from build123d import *

# Parameters (mm, degrees)
F0_W     = 127
F0_H     = 90.9382707423
F1_DEPTH = 76.2
F2_W     = 62.1625276506
F2_H     = 90.9382707423
F4_ANGLE = 45
F5_R     = 9.1670821984
F6_DEPTH = 114.3
F7_R     = 6.35


with BuildPart() as f1:
    # F0 (on Top) → F1 (new body)
    with BuildSketch(Plane.XY):
        with Locations((1.3374723494, 2.0061992109)):
            Rectangle(F0_W, F0_H)
    extrude(amount=F1_DEPTH)

    # F2 (on face) → F4 (revolve)
    with BuildSketch(Plane.XY.offset(76.2)):
        with Locations((-31.0812638253, 2.0061992109)):
            Rectangle(F2_W, F2_H)
    revolve(axis=Axis((0, 2.0061992109, 76.2), (0, 1, 0)), revolution_arc=F4_ANGLE)

    # F5 (on face) → F6 (join)
    with BuildSketch(Plane.XY.offset(76.2)):
        with Locations((35.0989550352, -15.1951536536)):
            Circle(F5_R)
    extrude(amount=F6_DEPTH)

    # F7
    f7_edges = [f1.edges().sort_by_distance(p)[0] for p in [
        (-43.955545, 2.006199, 120.155545),
    ]]
    fillet(f7_edges, radius=F7_R)


solid = f1.part
CAD build for the part. Positions are in the model's coordinates, mm. Round coordinates to 2 decimals unless told otherwise and drop trailing zeros. Order: outer loops, then holes, each group sorted by start corner. A loop starts at its lowest first (then second) coordinate and runs counter-clockwise, first axis right, second up. Notation, with made-up numbers: (-38.5, 25) - (-34.5, 25) arc R14 ccw to (-34.5, 46) - close; hole circle Ø5 at (63.25, 34.25). An arc over 180 degrees is marked (long way). Return JSON: item names as keys, results as strings.
(1) Cut at C-C (x = -27). Give the cut face in (y, z).
Answer key:
{"outline": "(-43.46, 0) - (47.48, 0) - (47.48, 103.2) - (-43.46, 103.2) - close"}
(2) Pin check, flat tips, straight feed: pin 1 Ø6 at (x, y) = (4, 28.5) entering from +Z; pin 2 Ø1.5 at (x, z) = (43, 135) entering from -Y; pin 3 Ø10 at (x, z) = (38, 120) entering from -Y. Stop position of each tip, or through.
Answer key:
{"pin 1": "stops at z = 76.2", "pin 2": "stops at y = -20.93", "pin 3": "stops at y = -24.36"}
(3) Pull direction X, two halves, no side cores. Call faces 1 (the face through (27.82, -20.77, 132.55)), 2 (the face through (64.837, 1, 38)), 3 (the face through (-58.79, 2.64, 96.4)), 4 (the face through (-19.9, 2.6, 96.1)): +X half, -X half, draft (parallel to the pull), parting line (faces both ways), or undercut.
Answer key:
{"face 1": "undercut", "face 2": "+X half", "face 3": "-X half", "face 4": "undercut"}
(4) Cut at D-D (y = -21). Give the cut face in (x, z), then the cut area to 3 significant figures.
Answer key:
{"outline": "(-62.16, 0) - (64.84, 0) - (64.84, 76.2) - (42.19, 76.2) - (42.19, 190.5) - (28, 190.5) - (28, 76.2) - (0, 76.2) - (-39.21, 115.41) arc R6.35 ccw to (-48.67, 114.87) arc R62.16 ccw to (-62.16, 76.2) - close", "area": "12,800 mm^2"}
(5) Wall check: probe 1 along Z at (x, y) = (5, 7); probe 2 along X at (y, z) = (-18, 107.5); probe 3 along X at (y, z) = (-28, 114). Give the ranges that are in metal, low to high. Write a range as from..to.
Answer key:
{"probe 1": "z = 0..76.2", "probe 2": "x = -53.71..-31.3, 26.37..43.83", "probe 3": "x = -49.35..-37.8"}
(6) Cut at B-B (z = 85). Give the cut face in (x, y), then the cut area to 3 significant figures.
Answer key:
{"outline": "(-61.54, -43.46) - (-8.8, -43.46) - (-8.8, 47.48) - (-61.54, 47.48) - close; circle Ø18.33 at (35.1, -15.2)", "area": "5,060 mm^2"}
(7) Cut at A-A (y = 11). Give the cut face in (x, z).
Answer key:
{"outline": "(-62.16, 0) - (64.84, 0) - (64.84, 76.2) - (0, 76.2) - (-39.21, 115.41) arc R6.35 ccw to (-48.67, 114.87) arc R62.16 ccw to (-62.16, 76.2) - close"}
